Can you work these out from the model? Positions are in its coordinate system, mm. Face numbers are marked on the shaded views. A direction names the side the tool comes from. Round coordinates to 2 decimals unless told otherwise and drop trailing zeros. Order: outer loops, then holes, each group sorted by start corner. A loop starts at its lowest first (then second) coordinate and runs counter-clockwise, first axis right, second up. Notation, with made-up numbers: M 54,25.25 L 104,25.25 A26 cw 104,55.25 Z; hole C 3,1 d2. An arc over 180 degrees is marked long. Answer as a JSON object with one key per item and string values. Group by question number.
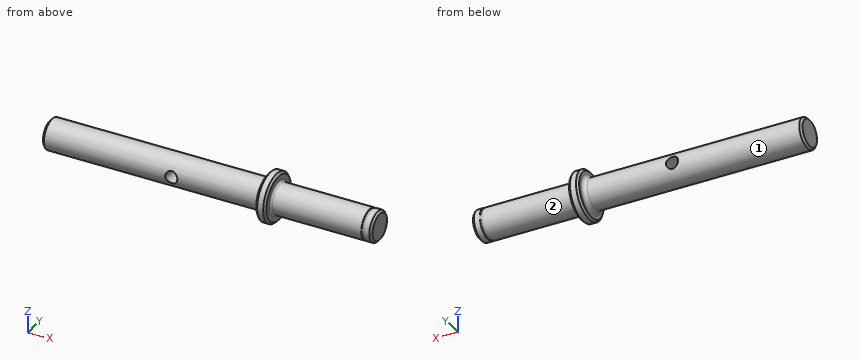
```python
from build123d import *

# Parameters (mm, degrees)
SKETCH2_R               = 3
CUT_EXTRUDE1_DEPTH      = 10
CUT_EXTRUDE1_DEPTH_BACK = 10
CHAMFER1_SIZE           = 1
FILLET1_R               = 2
FILLET2_R               = 1


with BuildPart() as part:
    # Sketch1 → Revolve1 (revolve)
    with BuildSketch(Plane.XY):
        Polygon((0, 0), (0, 7.5), (108, 7.5), (108, 12), (113, 12), (113, 7.5), (158, 7.5), (158, 7.15), (159.1, 7.15), (159.1, 7.5), (163, 7.5), (163, 0), align=None)
    revolve(axis=Axis((0, 0, 0), (-1, 0, 0)))

    # Sketch2 → Cut-Extrude1 (cut, two sides)
    with BuildSketch(Plane(origin=(0, 0, 0), x_dir=(1, 0, 0), z_dir=(0, 1, 0))) as cut_extrude1_sk:
        with Locations((64, 0)):
            Circle(SKETCH2_R)
    extrude(amount=CUT_EXTRUDE1_DEPTH, mode=Mode.SUBTRACT)
    extrude(cut_extrude1_sk.sketch, amount=-CUT_EXTRUDE1_DEPTH_BACK, mode=Mode.SUBTRACT)

    # Chamfer1
    chamfer1_edges = [part.edges().sort_by_distance(p)[0] for p in [
        (113, -12, 0),
        (108, -12, 0),
        (0, -7.5, 0),
        (163, -7.5, 0),
    ]]
    chamfer(chamfer1_edges, length=CHAMFER1_SIZE)

    # Fillet1
    fillet1_edges = [part.edges().sort_by_distance(p)[0] for p in [
        (108, -7.5, 0),
    ]]
    fillet(fillet1_edges, radius=FILLET1_R)

    # Fillet2
    fillet2_edges = [part.edges().sort_by_distance(p)[0] for p in [
        (113, -7.5, 0),
    ]]
    fillet(fillet2_edges, radius=FILLET2_R)


solid = part.part
```
1) For pin 1 (6 mm diameter, centred on x = 31.5, z = -1, fed in from -Y); pin 2 (4 mm diameter, centred on x = 78, z = -7, fed in from -Y); pin 3 (4 mm diameter, centred on x = 144.5, z = 1.5, fed in from +Y), each with a flat end and sliding along its axis, tell me the tip position at first contact or that it passes through.
2) If we section it at B-B on x = 64: Write out the boundary of the cut face in (y, z).
3) If we section it at A-A on x = 128.5: Write out the boundary of the cut face in (y, z), plus the area to 3 significant figures.
4) Which directions (+Z, -Z, +X, -X, +Y, -Y) give clear straight access to the entire face, cutting with the end or side of a thin tool? Please do the marked faces 1 and 2.
5) I need wall thicknesses on line 1 along X through (y, z) = (5.5, 0); line 2 along Z through (x, y) = (107, 4.25); line 3 along Z through (x, y) = (64, -3). Which ranges of each line are inside material? Lowest first, please.
Findings:
{
 "1": {"pin 1": "stops at y = -7.5", "pin 2": "stops at y = -5.59", "pin 3": "stops at y = 7.5"},
 "2": {"outline": "M -6.87,-3 A7.5 ccw 6.87,-3 Z; M -6.87,3 L 6.87,3 A7.5 ccw Z"},
 "3": {"outline": "C 0,0 d15", "area": "177 mm^2"},
 "4": {"face 1": "-X", "face 2": "+X"},
 "5": {"line 1": "x = 0 to 61, 67 to 163", "line 2": "z = -6.5 to 6.5", "line 3": "z = -6.87 to -3, 3 to 6.87"}
}
